Source: CAD feature listing. Evaluate the final solid. Frame: model axes, mm. A direction names the side the tool comes from. Round coordinates to 2 decimals unless told otherwise and drop trailing zeros. Write each loop counter-clockwise with the first axis right and the second up, starting at its lowest first coordinate (ties: lowest second). Pieces come first, ordered by that corner, then holes. Notation, with made-up numbers: M -39.75,42.25 L -26.75,42.25 A28 ccw -26.75,78.25 Z; hole C -6.5,-30 d1. An arc over 180 degrees is marked long. Use a Markdown table: item, result.
```python
from build123d import *

# Parameters (mm, degrees)
SKETCH1_W           = 165.1
SKETCH1_H           = 76.2
BOSS_EXTRUDE1_DEPTH = 3.175


with BuildPart() as part:
    # Sketch1 → Boss-Extrude1 (new body)
    with BuildSketch(Plane.XY):
        with Locations((9.351172696, -0.493343457)):
            Rectangle(SKETCH1_W, SKETCH1_H)
        with BuildLine():
            Line((51.769172696, 2.857146657), (51.769172696, -3.84383357))
            ThreePointArc((51.769172696, -3.84383357), (66.501172696, -0.493343457), (51.769172696, 2.857146657))
        make_face(mode=Mode.SUBTRACT)
        with BuildLine():
            Line((-27.798827304, 2.970758158), (-27.798827304, -3.957445072))
            ThreePointArc((-27.798827304, -3.957445072), (-47.798827304, -0.493343457), (-27.798827304, 2.970758158))
        make_face(mode=Mode.SUBTRACT)
        with BuildLine():
            Line((5.221172696, 2.970758158), (5.221172696, -3.957445072))
            ThreePointArc((5.221172696, -3.957445072), (-14.778827304, -0.493343457), (5.221172696, 2.970758158))
        make_face(mode=Mode.SUBTRACT)
        with BuildLine():
            Line((38.241172696, 2.970758158), (38.241172696, -3.957445072))
            ThreePointArc((38.241172696, -3.957445072), (18.241172696, -0.493343457), (38.241172696, 2.970758158))
        make_face(mode=Mode.SUBTRACT)
    extrude(amount=BOSS_EXTRUDE1_DEPTH)


solid = part.part
```
Q1. Section B-B on x = -44. Return loops of the section in (y, z) (3 decimals), plus the area to 3 significant figures.
Results are:
| item | result |
|---|---|
| outline | M -38.593,0 L -8.482,0 L -8.482,3.175 L -38.593,3.175 Z; M 7.496,0 L 37.607,0 L 37.607,3.175 L 7.496,3.175 Z |
| area | 191 mm^2 |
Q2. Reachability of faces 1 (the flat face through (91.901, -1, 2)), 2 (the flat face through (51.769, 0, 2)) from +Z, -Z, +X, -X, +Y, -Y: full face, straight path, thin tool, end or side. Return the list, or none.
Results are:
| item | result |
|---|---|
| face 1 | +Z, -Z, +X, +Y, -Y |
| face 2 | +Z, -Z |
Q3. Section A-A on z = 2.5. Return loops of the section in (x, y), plus the area to 3 significant figures.
Results are:
| item | result |
|---|---|
| outline | M -73.2,-38.59 L 91.9,-38.59 L 91.9,37.61 L -73.2,37.61 Z; hole M -27.8,-3.96 L -27.8,2.97 A10.3 ccw long Z; hole M 5.22,-3.96 L 5.22,2.97 A10.3 ccw long Z; hole M 38.24,-3.96 L 38.24,2.97 A10.3 ccw long Z; hole M 51.77,-3.84 A7.75 ccw long 51.77,2.86 Z |
| area | 11,400 mm^2 |
Q4. Section D-D on x = 1.5. Return loops of the section in (y, z) (3 decimals).
Results are:
| item | result |
|---|---|
| outline | M -38.593,0 L -8.88,0 L -8.88,3.175 L -38.593,3.175 Z; M 7.894,0 L 37.607,0 L 37.607,3.175 L 7.894,3.175 Z |
Q5. Mould query, pull axis X, two halves, no side actions, for faces 3 (the flat face through (-73.199, -1, 2)), 4 (the flat face through (8, 37.607, 2)), 5 (the flat face through (-27.799, 0, 2)). Classes: +X half, -X half, draft (parallel to the pull), parting line (faces both ways), or undercut.
Results are:
| item | result |
|---|---|
| face 3 | -X half |
| face 4 | draft |
| face 5 | undercut |
Q6. Line query: L1, parallel to X at y = -7.5, z = 0.65; L2, parallel to X at y = -4, z = 2.55; L3, parallel to Y at x = -30.5, z = 2.55. Output: solid intervals per line, ascending.
Results are:
| item | result |
|---|---|
| L1 | -73.2 to -45.05, -29.95 to -12.03, 3.07 to 20.99, 36.09 to 55.45, 62.06 to 91.9 |
| L2 | -73.2 to -47.18, -27.81 to -14.16, 5.21 to 18.86, 38.23 to 51.85, 65.66 to 91.9 |
| L3 | -38.59 to -8.05, 7.06 to 37.61 |
Q7. Section C-C on y = 5. Return loops of the section in (x, z) (3 decimals), plus the area to 3 significant figures.
Results are:
| item | result |
|---|---|
| outline | M -73.199,0 L -46.212,0 L -46.212,3.175 L -73.199,3.175 Z; M -28.786,0 L -13.192,0 L -13.192,3.175 L -28.786,3.175 Z; M 4.234,0 L 19.828,0 L 19.828,3.175 L 4.234,3.175 Z; M 37.254,0 L 53.292,0 L 53.292,3.175 L 37.254,3.175 Z; M 64.217,0 L 91.901,0 L 91.901,3.175 L 64.217,3.175 Z |
| area | 324 mm^2 |
